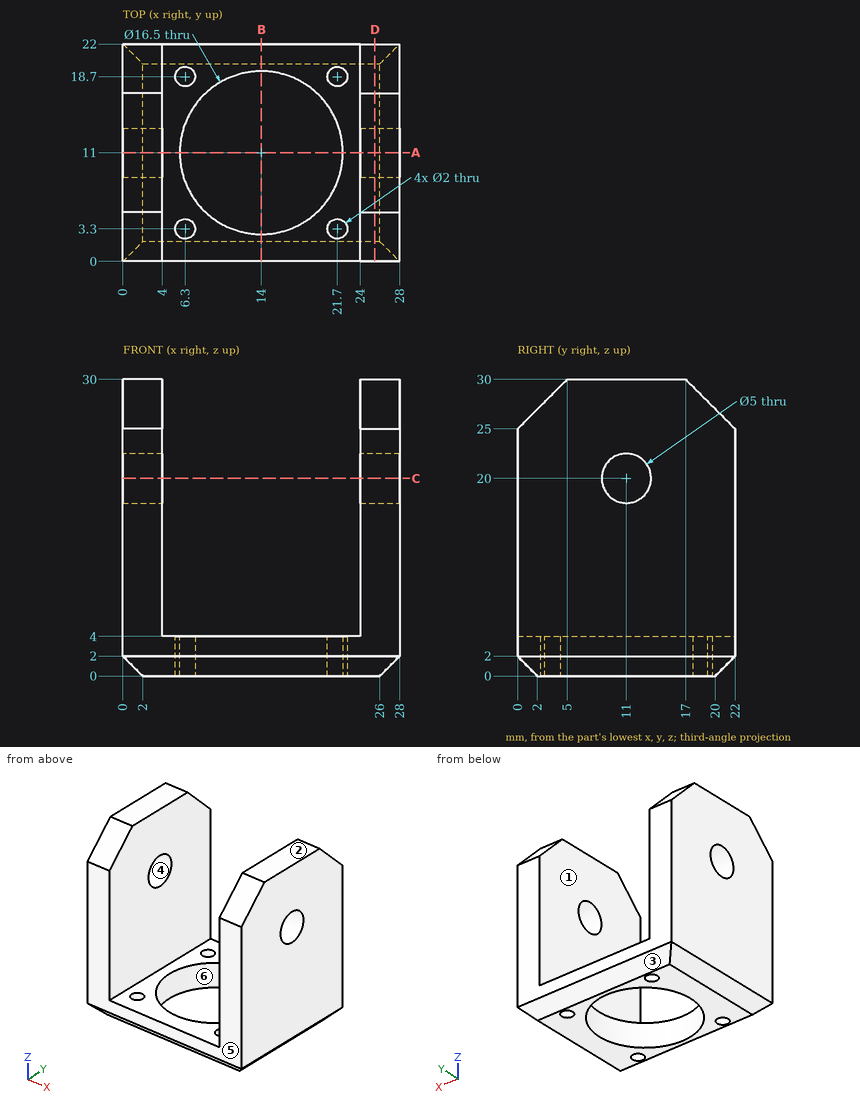
Answer from the drawing. Dimensions are ordinates in mm from the lowest x, y and z of the part. A direction names the side the tool comes from. Round coordinates to 2 decimals unless told otherwise and drop trailing zeros. Write each loop counter-clockwise with the first axis right and the second up, starting at its lowest first coordinate (ties: lowest second). Pieces come first, ordered by that corner, then holes. Notation, with made-up numbers: (-40, 80) - (-7, 80) arc R5 cw to (-7, 85) - close; hole circle Ø7 at (-13, 32). An arc over 180 degrees is marked (long way). Use a Markdown table: item, result.
(1) Which of the six approach directions +Z, -Z, +X, -X, +Y, -Y give full straight-line access (tool end or side, diameter ignored) to the marked faces 1 and 2?
Reported:
| item | result |
|---|---|
| face 1 | +Z, +Y, -Y |
| face 2 | +Z, +X, -X, +Y, -Y |
(2) This flat-tipped pin is pushed along its axis until it touches: pin 1 Ø10 at (x, y) = (13.5, 14.5) entering from +Z. Where does it stop, or does it pass through?
Reported:
| item | result |
|---|---|
| pin 1 | z = 4 |
(3) Straight lines are drawn through the part: line 1 along Y through (x, z) = (1.6, 20); line 2 along X through (y, z) = (10, 23); line 3 along Z through (x, y) = (22, 5.25). For each, find the intervals that lie inside material, in ascending order. Write a range as [from, to].
Reported:
| item | result |
|---|---|
| line 1 | [0, 8.5], [13.5, 22] |
| line 2 | [0, 4], [24, 28] |
| line 3 | [0, 4] |
(4) The part is cut by section C-C (z = 20). Write down the section's boundary in (x, y).
Reported:
| item | result |
|---|---|
| outline | (0, 0) - (4, 0) - (4, 8.5) - (0, 8.5) - close; (0, 13.5) - (4, 13.5) - (4, 22) - (0, 22) - close; (24, 0) - (28, 0) - (28, 8.5) - (24, 8.5) - close; (24, 13.5) - (28, 13.5) - (28, 22) - (24, 22) - close |
(5) The part is cut by section B-B (x = 14). Write down the section's boundary in (y, z), then the cut area to 3 significant figures.
Reported:
| item | result |
|---|---|
| outline | (0, 2) - (2, 0) - (2.75, 0) - (2.75, 4) - (0, 4) - close; (19.25, 0) - (20, 0) - (22, 2) - (22, 4) - (19.25, 4) - close |
| area | 18.0 mm2 |
(6) The part is cut by section A-A (y = 11). Write down the section's boundary in (x, z).
Reported:
| item | result |
|---|---|
| outline | (0, 2) - (2, 0) - (5.75, 0) - (5.75, 4) - (4, 4) - (4, 17.5) - (0, 17.5) - close; (0, 22.5) - (4, 22.5) - (4, 30) - (0, 30) - close; (22.25, 0) - (26, 0) - (28, 2) - (28, 17.5) - (24, 17.5) - (24, 4) - (22.25, 4) - close; (24, 22.5) - (28, 22.5) - (28, 30) - (24, 30) - close |
(7) The part is cut by section D-D (x = 25.5). Write down the section's boundary in (y, z), then the cut area to 3 significant figures.
Reported:
| item | result |
|---|---|
| outline | (0, 2) - (2, 0) - (20, 0) - (22, 2) - (22, 25) - (17, 30) - (5, 30) - (0, 25) - close; hole circle Ø5 at (11, 20) |
| area | 611 mm2 |
(8) The mould has two halves that part along Y. Classify the marked faces 3, 4, 5 and 6: released by +Y, released by -Y, zero draft, split by the parting line, or undercut.
Reported:
| item | result |
|---|---|
| face 3 | released by +Y |
| face 4 | undercut |
| face 5 | released by -Y |
| face 6 | undercut |
